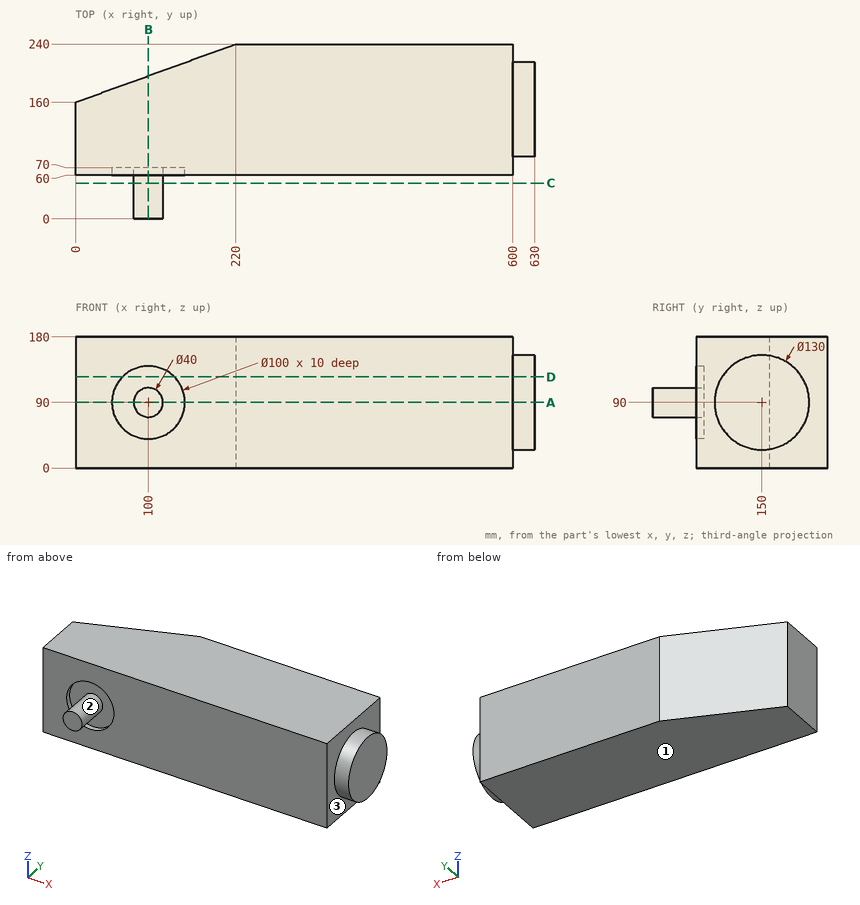
The drawing under review shows one solid part. Ordinate dimensions are in mm from its lowest x, y, z. A direction names the side the tool comes from. Coordinates: 2 decimals unless noted, no trailing zeros. Write each loop counter-clockwise with the first axis right and the second up, starting at its lowest first coordinate (ties: lowest second). Pieces come first, ordered by that corner, then holes. Notation, with made-up numbers: (77, 16) - (82, 16) arc R20 ccw to (82, 24) - close; hole circle Ø8 at (81, 25.25). An arc over 180 degrees is marked (long way). Answer in a Markdown table with one row per item. Add a question column.
Q1. For P1, Ø8, axis at x = 217.5, z = 137.5, coming from the -Y side; P2, Ø6, axis at y = 56, z = 100.5, coming from the +X side, all flat-tipped, find the tip position at first contact; note any pin that passes through.
Q2. For probe 1 along Z at (x, y) = (100, 63.25); probe 2 along X at (y, z) = (62, 78.5); probe 3 along Y at (x, z) = (592.5, 158), list the stretches that pass through material, from the lowest coordinate up.
Q3. We need section C-C, the plane y = 49. State the section outline as (x, z) points, and give its area (3 significant figures).
Q4. We need section A-A, the plane z = 90. State the section outline as (x, y) points, and give its area (3 significant figures).
Q5. Tool access review of the marked faces 1, 2 and 3: name each direction out of +Z, -Z, +X, -X, +Y, -Y from which nothing blocks a thin tool from reaching the whole face with its end or side.
Q6. We need section D-D, the plane z = 125. State the section outline as (x, y) points, and give its area (3 significant figures).
Q7. We need section B-B, the plane x = 100. State the section outline as (y, z) points.
Answer list:
| question | item | result |
|---|---|---|
| 1 | P1 | stops at y = 60 |
| 1 | P2 | stops at x = 118.54 |
| 2 | probe 1 | z = 0 to 40, 70 to 110, 140 to 180 |
| 2 | probe 2 | x = 0 to 51.34, 83.64 to 116.36, 148.66 to 600 |
| 2 | probe 3 | y = 60 to 240 |
| 3 | outline | circle Ø40 at (100, 90) |
| 3 | area | 1,260 mm2 |
| 4 | outline | (0, 60) - (50, 60) - (50, 70) - (80, 70) - (80, 0) - (120, 0) - (120, 70) - (150, 70) - (150, 60) - (600, 60) - (600, 85) - (630, 85) - (630, 215) - (600, 215) - (600, 240) - (220, 240) - (0, 160) - close |
| 4 | area | 105,000 mm2 |
| 5 | face 1 | -Z, +X, -X, +Y, -Y |
| 5 | face 2 | -Y |
| 5 | face 3 | +X |
| 6 | outline | (0, 60) - (64.29, 60) - (64.29, 70) - (135.71, 70) - (135.71, 60) - (600, 60) - (600, 95.23) - (630, 95.23) - (630, 204.77) - (600, 204.77) - (600, 240) - (220, 240) - (0, 160) - close |
| 6 | area | 102,000 mm2 |
| 7 | outline | (0, 70) - (70, 70) - (70, 40) - (60, 40) - (60, 0) - (196.36, 0) - (196.36, 180) - (60, 180) - (60, 140) - (70, 140) - (70, 110) - (0, 110) - close |
